```python
from build123d import *

# Parameters (mm, degrees)
BOSS_EXTRUDE1_START = 18
BOSS_EXTRUDE1_DEPTH = 18
BOSS_EXTRUDE2_DEPTH = 18
FILLET1_SIZE        = 2


with BuildPart() as part:
    # Sketch1 → Revolve1 (revolve)
    with BuildSketch(Plane.XY):
        Polygon((-9.207, 38), (-9.207, 0), (-5.207, 0), (-5.207, 18), (0, 18), (0, 20), (-4.2, 20), (-4.2, 38), align=None)
    revolve(axis=Axis((0, 38, 0), (0, -1, 0)))

    # Sketch3 → Boss-Extrude1 (add)
    with BuildSketch(Plane(origin=(0, 20, 0), x_dir=(1, 0, 0), z_dir=(0, 1, 0)).offset(BOSS_EXTRUDE1_START)):
        with BuildLine():
            Line((-2.5, 3.374907406), (-2.5, -3.374907406))
            ThreePointArc((-2.5, -3.374907406), (-4.2, 0), (-2.5, 3.374907406))
        make_face()
    extrude(amount=-BOSS_EXTRUDE1_DEPTH)

    # Sketch2 → Boss-Extrude2 (add)
    with BuildSketch(Plane.XZ.offset(-18)):
        with BuildLine():
            ThreePointArc((5.207, 0), (4.946482892, 1.626393556), (4.191, 3.090043365))
            Line((4.191, 3.090043365), (4.191, -3.090043365))
            ThreePointArc((4.191, -3.090043365), (4.946482892, -1.626393556), (5.207, 0))
        make_face()
    extrude(amount=BOSS_EXTRUDE2_DEPTH)

    # Fillet1
    # a fillet whose section is not a circle: 2 mm, written as the material it takes off along each edge
    with BuildSketch(Plane(origin=(0, 0, 0), x_dir=(-1, 0, 0), z_dir=(0, 0, 1))) as fillet1_piece_1:
        with BuildLine():
            add(Edge.make_bspline([(9.207, -FILLET1_SIZE), (9.207, -FILLET1_SIZE * 0.831801948466), (9.207, -FILLET1_SIZE * 0.663603896932), (9.207 - FILLET1_SIZE * 0.0716919198361, -FILLET1_SIZE * 0.292893218813), (9.207 - FILLET1_SIZE * 0.292893218813, -FILLET1_SIZE * 0.0716919198361), (9.207 - FILLET1_SIZE * 0.663603896932, 0), (9.207 - FILLET1_SIZE * 0.831801948466, 0), (9.207 - FILLET1_SIZE, 0)], knots=[0, 0, 0, 0, 0, 0, 0.5, 0.5, 1, 1, 1, 1, 1, 1], degree=5))
            Line((9.207 - FILLET1_SIZE, 0), (9.207, 0))
            Line((9.207, 0), (9.207, -FILLET1_SIZE))
        make_face()
    revolve(axis=Axis((0, 0, 0), (0, -1, 0)), mode=Mode.SUBTRACT)
    with BuildSketch(Plane(origin=(0, 38, 0), x_dir=(-1, 0, 0), z_dir=(0, 0, 1))) as fillet1_piece_2:
        with BuildLine():
            add(Edge.make_bspline([(9.207, FILLET1_SIZE), (9.207, FILLET1_SIZE * 0.831801948466), (9.207, FILLET1_SIZE * 0.663603896932), (9.207 - FILLET1_SIZE * 0.0716919198361, FILLET1_SIZE * 0.292893218813), (9.207 - FILLET1_SIZE * 0.292893218813, FILLET1_SIZE * 0.0716919198361), (9.207 - FILLET1_SIZE * 0.663603896932, 0), (9.207 - FILLET1_SIZE * 0.831801948466, 0), (9.207 - FILLET1_SIZE, 0)], knots=[0, 0, 0, 0, 0, 0, 0.5, 0.5, 1, 1, 1, 1, 1, 1], degree=5))
            Line((9.207 - FILLET1_SIZE, 0), (9.207, 0))
            Line((9.207, 0), (9.207, FILLET1_SIZE))
        make_face()
    revolve(axis=Axis((0, 38, 0), (0, -1, 0)), mode=Mode.SUBTRACT)


solid = part.part
```
Geometry: final body of the model. Coordinates: model frame, mm. A direction names the side the tool comes from. Give positions to 0.01 mm unless a question says otherwise; leave off trailing zeros. Loops run counter-clockwise (first coordinate to the right, second up) from the corner with the lowest first, then second, coordinate; pieces in that order, holes last. Notation, with made-up numbers: (10, 78.5) -> (36, 78.5) arc R20 cw to (36, 95.5) -> close; hole circle Ø7 at (85.25, 8.5). An arc over 180 degrees is marked (long way). Use CSV: the item, a comma, the result in double quotes.
(1) Cut plane B-B (y = 33). Output: boundary loops of the cut face in (x, z), plus the area to 3 significant figures.
From the geometry:
outline,"circle Ø18.41 at (0, 0); hole (-2.5, -3.37) arc R4.2 ccw (long way) to (-2.5, 3.37) -> close"
area,"219 mm^2"
(2) Access query for faces 4 (the face through (1, 20, 0)), 5 (the face through (4.191, 9, 0)), 6 (the face through (-3, 38, 0)). Directions: +Z, -Z, +X, -X, +Y, -Y. A direction counts if a zero-diameter tool reaches every point of the face in a straight line with its end or side. Return the directions, or none.
From the geometry:
face 4,"+Y"
face 5,"-Y"
face 6,"+Z, -Z, +X, -X, +Y"
(3) Ray query, line 1 along Z through (x, y) = (0, 5); line 2 along X through (y, z) = (5, 0); line 3 along X through (y, z) = (35, -0.25). Return the intervals inside material, ascending. Write a range as [from, to].
From the geometry:
line 1,"[-9.21, -5.21], [5.21, 9.21]"
line 2,"[-9.21, -5.21], [4.19, 9.21]"
line 3,"[-9.2, -2.5], [4.19, 9.2]"
(4) First-contact query: P1, Ø4, axis at x = -2, z = 0.5, coming from the -Y side; P2, Ø8, axis at y = 23.5, z = -7, coming from the +X side; P3, Ø3, axis at y = 9, z = 5, coming from the +X side. Flat tips, straight axial feed; report the tip coordinate or a pass-through.
From the geometry:
P1,"y = 18"
P2,"x = 8.7"
P3,"x = 8.52"
(5) Cut plane A-A (y = 15). Output: boundary loops of the cut face in (x, z), plus the area to 3 significant figures.
From the geometry:
outline,"circle Ø18.41 at (0, 0); hole (4.19, -3.09) -> (4.19, 3.09) arc R5.21 ccw (long way) to start"
area,"185 mm^2"
(6) Pull-direction query (X, two-part tool) for faces 1 (the face through (-2.5, 29, 0)), 2 (the face through (7.31, 18.76, 5.6)), 3 (the face through (5, 0, 0)); classes: released by +X, released by -X, zero draft, split by the parting line, or undercut.
From the geometry:
face 1,"undercut"
face 2,"split by the parting line"
face 3,"zero draft"
